from build123d import *

# Parameters (mm, degrees)
F0_R      = 25.4
F1_DEPTH  = 6.35
F2_R      = 22.225
F3_DEPTH  = 12.7
F4_R      = 25.4
F4_R_2    = 22.225
F5_DEPTH  = 6.35
F7_D      = 3.175
F7_DEPTH  = 3.175
F7_TIP    = 0.9538662327
F8_D      = 12.7
F9_R      = 1.58749
F10_DEPTH = 6.35


# Not quite as in the source:
# - a fillet or chamfer is up to 0.001 mm smaller than in the source, because OpenCascade refuses the exact size


with BuildPart() as f1:
    # F0 (on Front) → F1 (new body)
    with BuildSketch(Plane.XZ):
        with Locations((0, -3.2290907108)):
            Circle(F0_R)
    extrude(amount=F1_DEPTH)

    # F2 (on face) → F3 (join)
    with BuildSketch(Plane.XZ.offset(6.35)):
        with Locations((0, -3.2290907108)):
            Circle(F2_R)
    extrude(amount=F3_DEPTH)

    # F4 (on face) → F5 (join)
    with BuildSketch(Plane.XZ.offset(19.05)):
        with Locations((0, -3.2290907108)):
            Circle(F4_R)
        with Locations((0, -3.2290907108)):
            Circle(F4_R_2, mode=Mode.SUBTRACT)
        with Locations((0, -3.2290907108)):
            Circle(F4_R_2)
    extrude(amount=F5_DEPTH)

    # F7
    with Locations(Plane.XZ.offset(25.4)):
        with Locations((19.05, -3.2290907108), (0, -22.2790907108), (-19.05, -3.2290907108), (0, 15.8209092892)):
            Hole(F7_D / 2, depth=F7_DEPTH)
            with Locations((0, 0, -(F7_DEPTH + F7_TIP / 2))):  # 118° drill point
                Cone(0, F7_D / 2, F7_TIP, mode=Mode.SUBTRACT)

    # F8 (through all)
    with Locations(Plane(origin=(0, 0, 0), x_dir=(1, 0, 0), z_dir=(0, 1, 0))):
        with Locations((0, 3.2290907108)):
            Hole(F8_D / 2)

    # F9 (radius 1.5875 in the source; OpenCascade refuses exactly that, so slightly less here)
    f9_edges = [f1.edges().sort_by_distance(p)[0] for p in [
        (-25.4, -6.35, -3.229091),
        (-25.4, 0, -3.229091),
        (-22.225, -6.35, -3.229091),
        (-25.4, -25.4, -3.229091),
        (-25.4, -19.05, -3.229091),
        (-22.225, -19.05, -3.229091),
    ]]
    fillet(f9_edges, radius=F9_R)

    # F4 (on face) → F10 (join)
    with BuildSketch(Plane.XZ.offset(19.05)):
        with Locations((0, -3.2290907108)):
            Circle(F4_R)
    extrude(amount=F10_DEPTH)


solid = f1.part
The model under review builds one solid part; all positions refer to its coordinate system, in mm. A direction names the side the tool comes from. Round coordinates to 2 decimals unless told otherwise and drop trailing zeros. Loops run counter-clockwise (first coordinate to the right, second up) from the corner with the lowest first, then second, coordinate; pieces in that order, holes last. Notation, with made-up numbers: (-21, 22) -> (38, 22) arc R30 ccw to (38, 46) -> close; hole circle Ø4 at (11.5, 74). An arc over 180 degrees is marked (long way). Return JSON: item names as keys, results as strings.
(1) Add section C-C on y = -22.75. Write out the cut boundary in (x, z), plus the area to 3 significant figures.
Solved:
{"outline": "circle Ø50.8 at (0, -3.23)", "area": "2,030 mm2"}
(2) For faces 1 (the cylindrical face through (-17.6, -12.6, -16.8)), 2 (the flat face through (5, 0, -8)), list the 3-axis set-ups (+Z, -Z, +X, -X, +Y, -Y) from which the entire face can be reached by the end or side of a thin tool; tool diameter is ignored.
Solved:
{"face 1": "none", "face 2": "+Z, -Z, +X, -X, +Y"}
(3) Add section D-D on y = -9. Write out the cut boundary in (x, z) (3 decimals).
Solved:
{"outline": "circle Ø44.45 at (0, -3.229); hole circle Ø12.7 at (0, -3.229)"}
(4) For pin 1 (3 mm diameter, centred on x = 19.5, y = -14, fed in from +Z); pin 2 (8 mm diameter, centred on x = 17.5, y = -9.5, fed in from +Z); pin 3 (6 mm diameter, centred on x = -18.5, y = -19, fed in from +Z), all flat-tipped, find the tip position at first contact; note any pin that passes through.
Solved:
{"pin 1": "z = 9.81", "pin 2": "z = 16.09", "pin 3": "z = 16.89"}
(5) Add section B-B on y = -5.5. Write out the cut boundary in (x, z), plus the area to 3 significant figures.
Solved:
{"outline": "circle Ø50.44 at (0, -3.23); hole circle Ø12.7 at (0, -3.23)", "area": "1,870 mm2"}
(6) For line 1 (Z direction, x = 0, y = -4.75); line 2 (Z direction, x = 0, y = -11); line 3 (X direction, y = -7.5, z = -1), list the stretches that pass through material, from the lowest coordinate up.
Solved:
{"line 1": "-28.63 to -9.58, 3.12 to 22.17", "line 2": "-25.45 to -9.58, 3.12 to 19", "line 3": "-22.17 to -5.95, 5.95 to 22.17"}
(7) The part is to be moulded in two halves that separate along Z. For faces 3 (the cylindrical face through (1.38, -9.66, 2.97)), 4 (the flat face through (-23, -19.05, -11)), 5 (the cylindrical face through (-20.16, -3.15, -18.68)), 6 (the flat face through (0, -19.05, -3)), say which applies: released by +Z, released by -Z, zero draft, split by the parting line, or undercut.
Solved:
{"face 3": "undercut", "face 4": "zero draft", "face 5": "split by the parting line", "face 6": "undercut"}
